Can you work these out from the model? Positions are in its coordinate system, mm. A direction names the side the tool comes from. Give positions to 0.01 mm unless a question says otherwise; leave off trailing zeros. Write each loop counter-clockwise with the first axis right and the second up, starting at its lowest first coordinate (ties: lowest second). Pieces come first, ordered by that corner, then holes. Notation, with made-up numbers: (76, 63.5) - (123, 63.5) arc R14 ccw to (123, 79.5) - close; hole circle Ø1 at (81.25, 46). An arc over 180 degrees is marked (long way). Return JSON: item names as keys, results as strings. Group by question number.
from build123d import *

# Parameters (mm, degrees)
BOSS_EXTRUDE1_DEPTH = 31.75


with BuildPart() as part:
    # Sketch1 → Boss-Extrude1 (new body)
    with BuildSketch(Plane.XY):
        with BuildLine():
            Line((-2.670777087, -1.016), (-9.020777087, -1.016))
            Line((-9.020777087, -1.016), (-9.020777087, -2.032))
            Line((-9.020777087, -2.032), (-2.032, -2.032))
            Line((-2.032, -2.032), (-1.122532015, -1.122532015))
            ThreePointArc((-1.122532015, -1.122532015), (0, 1.5875), (1.122532015, -1.122532015))
            Line((1.122532015, -1.122532015), (2.032, -2.032))
            Line((2.032, -2.032), (9.020777087, -2.032))
            Line((9.020777087, -2.032), (9.020777087, -1.016))
            Line((9.020777087, -1.016), (2.670777087, -1.016))
            ThreePointArc((2.670777087, -1.016), (0, 2.8575), (-2.670777087, -1.016))
        make_face()
    extrude(amount=BOSS_EXTRUDE1_DEPTH)


solid = part.part
1) Will these pins go through, and if not, where does the flat tip stop? pin 1 Ø2 at (x, z) = (4, 12) entering from +Y; pin 2 Ø1 at (y, z) = (1.5, 11) entering from -X; pin 3 Ø1.5 at (y, z) = (2.5, 4) entering from +X.
2) On a 3-axis mill with a long thin cutter (end or side, diameter ignored), from which of +Z, -Z, +X, -X, +Y, -Y can I reach the whole of each face in a straight line? I mean faces 5 (the face through (-9.021, -1.5, 15.7)), 6 (the face through (1.6, -1.6, 15.7)). Say none if no direction works.
3) I need wall thicknesses on line 1 along X through (y, z) = (0, 11); line 2 along Y through (x, z) = (0, 7.5); line 3 along Y through (x, z) = (4.25, 3). Which ranges of each line are inside material? Lowest first, please.
4) Imagine slicing it at A-A, the plane y = 0. Write out the boundary of the cut face in (x, z), and give its area (3 significant figures).
5) Imagine slicing it at B-B, the plane z = 7. Write out the boundary of the cut face in (x, y) (1 decimal).
6) We'd pull the mould along Y, two halves only. Please class faces 1 (the face through (0.077, 2.856, 15.653)), 2 (the face through (-0.052, 1.587, 15.653)), 3 (the face through (5, -2.032, 16)), 4 (the face through (9.021, -1.5, 15.7)): pulls with the +Y half, pulls with the -Y half, needs draft (parallel to the pull), parting line crosses it, or undercut.
7) Imagine slicing it at D-D, the plane x = 0. Write out the boundary of the cut face in (y, z).
8) Imagine slicing it at C-C, the plane y = -1.5. Write out the boundary of the cut face in (x, z).
Resolved:
{
 "1": {"pin 1": "y = -1.02", "pin 2": "x = -2.68", "pin 3": "x = 2.26"},
 "2": {"face 5": "+Z, -Z, -X, +Y, -Y", "face 6": "+Z, -Z, -Y"},
 "3": {"line 1": "-2.86 to -1.59, 1.59 to 2.86", "line 2": "1.59 to 2.86", "line 3": "-2.03 to -1.02"},
 "4": {"outline": "(-2.86, 0) - (-1.59, 0) - (-1.59, 31.75) - (-2.86, 31.75) - close; (1.59, 0) - (2.86, 0) - (2.86, 31.75) - (1.59, 31.75) - close", "area": "80.6 mm^2"},
 "5": {"outline": "(-9, -2) - (-2, -2) - (-1.1, -1.1) arc R1.6 cw (long way) to (1.1, -1.1) - (2, -2) - (9, -2) - (9, -1) - (2.7, -1) arc R2.9 ccw (long way) to (-2.7, -1) - (-9, -1) - close"},
 "6": {"face 1": "undercut", "face 2": "undercut", "face 3": "pulls with the -Y half", "face 4": "needs draft"},
 "7": {"outline": "(1.59, 0) - (2.86, 0) - (2.86, 31.75) - (1.59, 31.75) - close"},
 "8": {"outline": "(-9.02, 0) - (-1.5, 0) - (-1.5, 31.75) - (-9.02, 31.75) - close; (1.5, 0) - (9.02, 0) - (9.02, 31.75) - (1.5, 31.75) - close"}
}
